Work out the finished part from the listing and answer in its coordinate system (mm). Face numbers are marked on the shaded views. Coordinates: 2 decimals unless noted, no trailing zeros. Write each loop counter-clockwise with the first axis right and the second up, starting at its lowest first coordinate (ties: lowest second). Pieces come first, ordered by that corner, then holes. Notation, with made-up numbers: (-2.75, 46) - (28.25, 46) arc R33 ccw to (28.25, 76) - close; hole circle Ø5 at (-17.5, -35.5). An arc over 180 degrees is marked (long way). Use a Markdown table: item, result. Add a question column.
(1) Given pin 1 Ø8 at (x, y) = (0, 0) entering from -Z; pin 2 Ø10 at (x, y) = (0.5, 0.5) entering from +Z, each flat-ended and moving along its own axis, determine where each tip first touches the part or whether it passes through.
(2) Find the intervals of material crossed by line 1 (Z direction, x = -4.5, y = -7.5); line 2 (Y direction, x = 9, z = 2.9); line 3 (Y direction, x = 6.25, z = 4.65), in increasing order. Write a range as from..to.
(3) For a pull along Z with two mould halves and no side action, classify the marked faces 1, 2, 3 and 4 as released by +Z, released by -Z, zero draft, split by the parting line, or undercut.
(4) The part is cut by section A-A, the plane x = 0. Give the vertices of the cut face in (y, z).
from build123d import *

# Parameters (mm, degrees)
F0_R          = 11
F0_R_2        = 10.5
F0_R_3        = 10.05
F1_DEPTH      = 5
F4_R          = 11
F4_R_2        = 10.5
F5_DEPTH      = 2
F5_DEPTH_BACK = 1
F0_R_4        = 4.5
F9_DEPTH      = 0.5
F0_R_5        = 3.5
F10_DEPTH     = 1


# Not quite as in the source:
# - a fillet or chamfer that OpenCascade refuses, or shapes differently, is made with other operations: its cross-section is extruded or revolved along the edge and cut away or added


with BuildPart() as f1:
    # F0 (on Top) → F1 (new body)
    with BuildSketch(Plane.XY):
        Circle(F0_R)
        Circle(F0_R_2, mode=Mode.SUBTRACT)
        Circle(F0_R_2)
        Circle(F0_R_3, mode=Mode.SUBTRACT)
    extrude(amount=F1_DEPTH)

    # F4 (on plane+point) → F5 (cut, two sides)
    with BuildSketch(Plane.XY.offset(2.5)) as f5_sk:
        Circle(F4_R)
        Circle(F4_R_2, mode=Mode.SUBTRACT)
    extrude(amount=-F5_DEPTH, mode=Mode.SUBTRACT)
    extrude(f5_sk.sketch, amount=F5_DEPTH_BACK, mode=Mode.SUBTRACT)

    # F6: chamfer of 1 on 1 edges, made by hand

    # F6_s1 → F6_t2 (revolve, cut)
    with BuildSketch(Plane.XZ):
        Polygon((11, 4), (10, 5), (11, 5), align=None)
    revolve(axis=Axis((0, 0, 5), (0, 0, 1)), mode=Mode.SUBTRACT)

    # F7: fillet of radius 1 on 2 edges, made by hand

    # F7_s1 → F7_t2 (revolve)
    with BuildSketch(Plane.XZ):
        with BuildLine():
            ThreePointArc((10.5, 2.6339745962), (10.6339745962, 3.1339745962), (11, 3.5))
            Line((11, 3.5), (10.5, 3.5))
            Line((10.5, 3.5), (10.5, 2.6339745962))
        make_face()
    revolve(axis=Axis((0, 0, 3.5), (0, 0, 1)))

    # F7_s3 → F7_t4 (revolve)
    with BuildSketch(Plane.XZ):
        with BuildLine():
            ThreePointArc((11, 0.5), (10.6339745962, 0.8660254038), (10.5, 1.3660254038))
            Line((10.5, 1.3660254038), (10.5, 0.5))
            Line((10.5, 0.5), (11, 0.5))
        make_face()
    revolve(axis=Axis((0, 0, 0.5), (0, 0, 1)))

    # F8: chamfer of 1 on 2 edges, made by hand

    # F8_s1 → F8_t2 (revolve, cut)
    with BuildSketch(Plane.XZ):
        with BuildLine():
            Line((10.6709126952, 3.1725042869), (11.0121000067, 4.2475531418))
            Line((11.0121000067, 4.2475531418), (11.0321000067, 4.2475531418))
            ThreePointArc((11.0321000067, 4.2475531418), (11.02, 3.8737765709), (11.02, 3.5))
            Line((11.02, 3.5), (11.01, 3.4826794919))
            ThreePointArc((11.01, 3.4826794919), (10.8264226951, 3.3457987418), (10.6872524412, 3.1609711736))
            Line((10.6872524412, 3.1609711736), (10.6709126952, 3.1725042869))
        make_face()
    revolve(axis=Axis((0, 0, 3.5), (0, 0, 1)), mode=Mode.SUBTRACT)

    # F8_s3 → F8_t4 (revolve, cut)
    with BuildSketch(Plane.XZ):
        with BuildLine():
            Line((11.0121000067, -0.2475531418), (10.6709126952, 0.8274957131))
            Line((10.6709126952, 0.8274957131), (10.6872524412, 0.8390288264))
            ThreePointArc((10.6872524412, 0.8390288264), (10.8264226951, 0.6542012582), (11.01, 0.5173205081))
            Line((11.01, 0.5173205081), (11.02, 0.5))
            ThreePointArc((11.02, 0.5), (11.02, 0.1262234291), (11.0321000067, -0.2475531418))
            Line((11.0321000067, -0.2475531418), (11.0121000067, -0.2475531418))
        make_face()
    revolve(axis=Axis((0, 0, 0.5), (0, 0, 1)), mode=Mode.SUBTRACT)

    # F0 (on Top) → F9 (join)
    with BuildSketch(Plane.XY):
        Circle(F0_R_3)
        Circle(F0_R_4, mode=Mode.SUBTRACT)
    extrude(amount=F9_DEPTH)

    # F0 (on Top) → F10 (join)
    with BuildSketch(Plane.XY):
        Circle(F0_R_4)
        Circle(F0_R_5, mode=Mode.SUBTRACT)
    extrude(amount=F10_DEPTH)


solid = f1.part
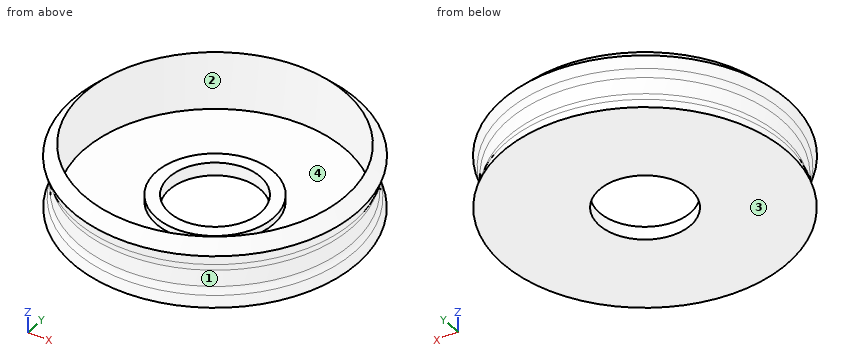
Model answer:
| question | item | result |
|---|---|---|
| 1 | pin 1 | z = 0 |
| 1 | pin 2 | z = 1 |
| 2 | line 1 | 0..0.5 |
| 2 | line 2 | -5.48..-4.47, 4.47..5.48 |
| 2 | line 3 | -8.25..-7.87, 7.87..8.25 |
| 3 | face 1 | undercut |
| 3 | face 2 | zero draft |
| 3 | face 3 | released by -Z |
| 3 | face 4 | released by +Z |
| 4 | outline | (-10.95, 4.05) - (-10.68, 3.21) arc R1 cw to (-10.5, 2.63) - (-10.5, 1.37) arc R1 cw to (-10.68, 0.79) - (-10.93, 0) - (-3.5, 0) - (-3.5, 1) - (-4.5, 1) - (-4.5, 0.5) - (-10.05, 0.5) - (-10.05, 4.95) - close; (3.5, 0) - (10.93, 0) - (10.68, 0.79) arc R1 cw to (10.5, 1.37) - (10.5, 2.63) arc R1 cw to (10.68, 3.21) - (10.95, 4.05) - (10.05, 4.95) - (10.05, 0.5) - (4.5, 0.5) - (4.5, 1) - (3.5, 1) - close |
